Part print with two shaded views. Sizes in mm from the minimum x, y, z corner. A direction names the side the tool comes from. Give positions to 0.01 mm unless a question says otherwise; leave off trailing zeros. Loops run counter-clockwise (first coordinate to the right, second up) from the corner with the lowest first, then second, coordinate; pieces in that order, holes last. Notation, with made-up numbers: M 46.25,55 L 50.25,55 A21 cw 50.25,80 Z; hole C -4,7 d8. An arc over 180 degrees is marked long. Answer in a Markdown table with one row per item.
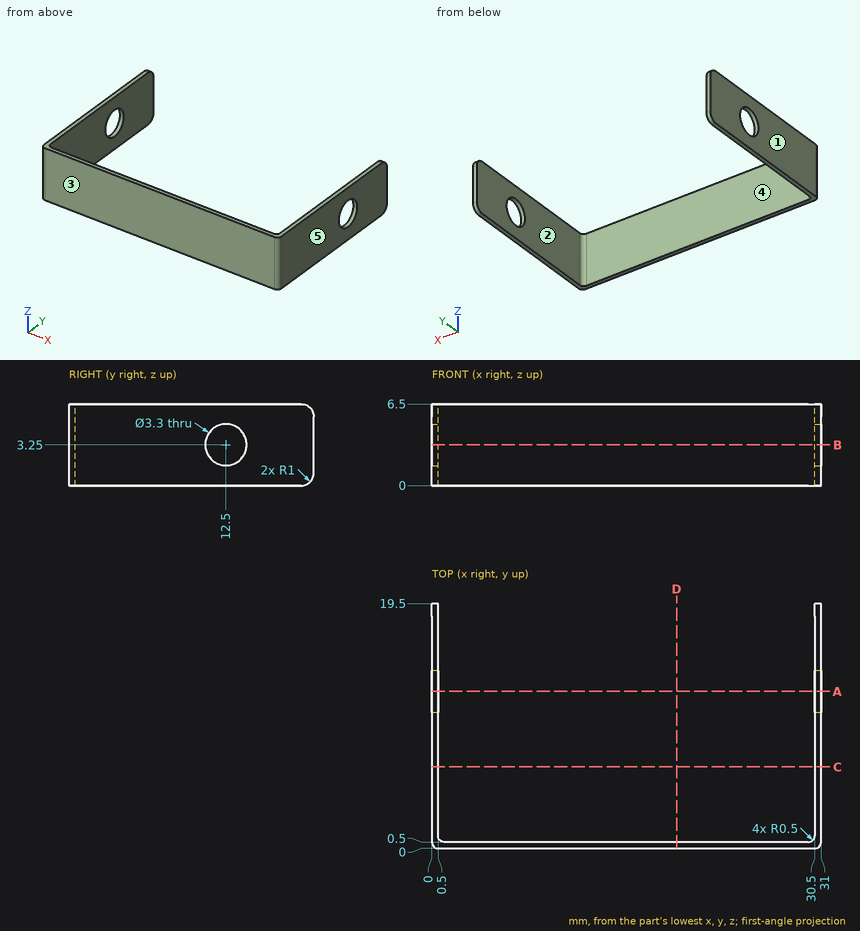
Q1. Drop flat-ended pins along their axis: pin 1 (3 mm diameter, centred on x = 3.5, z = 2, fed in from +Y); pin 2 (3 mm diameter, centred on y = 12.5, z = 3.25, fed in from +X). Give the stop position or say it passes through.
Reported:
| item | result |
|---|---|
| pin 1 | y = 0.5 |
| pin 2 | through |
Q2. Saw through at C-C (y = 6.5). Give the cut face in (x, z), and give its area (3 significant figures).
Reported:
| item | result |
|---|---|
| outline | M 0,0 L 0.5,0 L 0.5,6.5 L 0,6.5 Z; M 30.5,0 L 31,0 L 31,6.5 L 30.5,6.5 Z |
| area | 6.50 mm² |
Q3. 3-axis set-ups, long thin cutter, end or side, ignore diameter. For the marked faces 4 and 5: which of +Z, -Z, +X, -X, +Y, -Y reach the whole face in a straight line?
Reported:
| item | result |
|---|---|
| face 4 | +Z, -Z, +Y |
| face 5 | +Z, -Z, +X, +Y, -Y |
Q4. Probe probe 1 along X at (y, z) = (14.25, 4.25); probe 2 along Z at (x, y) = (30.75, 12.5); probe 3 along Y at (x, z) = (23.5, 3.5). List the from-to ranges inside material, lowest first.
Reported:
| item | result |
|---|---|
| probe 1 | 0 to 0.5, 30.5 to 31 |
| probe 2 | 0 to 1.6, 4.9 to 6.5 |
| probe 3 | 0 to 0.5 |
Q5. Saw through at D-D (x = 19.5). Give the cut face in (y, z).
Reported:
| item | result |
|---|---|
| outline | M 0,0 L 0.5,0 L 0.5,6.5 L 0,6.5 Z |
Q6. Mould opens along X. For the marked faces 1, 2 and 3 say: released by +X, released by -X, zero draft, split by the parting line, or undercut.
Reported:
| item | result |
|---|---|
| face 1 | released by -X |
| face 2 | undercut |
| face 3 | zero draft |
Q7. Saw through at B-B (z = 3.25). Give the cut face in (x, y), and give its area (3 significant figures).
Reported:
| item | result |
|---|---|
| outline | M 0,0.5 A0.5 ccw 0.5,0 L 30.5,0 A0.5 ccw 31,0.5 L 31,10.85 L 30.5,10.85 L 30.5,1 A0.5 cw 30,0.5 L 1,0.5 A0.5 cw 0.5,1 L 0.5,10.85 L 0,10.85 Z; M 0,14.15 L 0.5,14.15 L 0.5,19.5 L 0,19.5 Z; M 30.5,14.15 L 31,14.15 L 31,19.5 L 30.5,19.5 Z |
| area | 31.2 mm² |
Q8. Saw through at A-A (y = 12.5). Give the cut face in (x, z), and give its area (3 significant figures).
Reported:
| item | result |
|---|---|
| outline | M 0,0 L 0.5,0 L 0.5,1.6 L 0,1.6 Z; M 0,4.9 L 0.5,4.9 L 0.5,6.5 L 0,6.5 Z; M 30.5,0 L 31,0 L 31,1.6 L 30.5,1.6 Z; M 30.5,4.9 L 31,4.9 L 31,6.5 L 30.5,6.5 Z |
| area | 3.20 mm² |
